```python
from build123d import *

# Parameters (mm, degrees)
SKETCH2_W           = 57.15
SKETCH2_H           = 184.15
BOSS_EXTRUDE1_DEPTH = 6.35
SKETCH3_W           = 44.45
SKETCH3_H           = 6.985
CUT_EXTRUDE1_DEPTH  = 97.616037747
SKETCH4_W           = 6.985
SKETCH4_H           = 50.8
CUT_EXTRUDE2_DEPTH  = 97.616037747


with BuildPart() as part:
    # Sketch2 → Boss-Extrude1 (new body)
    with BuildSketch(Plane.XY):
        Rectangle(SKETCH2_W, SKETCH2_H)
    extrude(amount=BOSS_EXTRUDE1_DEPTH)

    # Sketch3 → Cut-Extrude1 (cut, through all)
    with BuildSketch(Plane.XY.offset(6.35)):
        with Locations((0, 82.2325)):
            Rectangle(SKETCH3_W, SKETCH3_H)
    extrude(amount=-CUT_EXTRUDE1_DEPTH, mode=Mode.SUBTRACT)

    # Sketch4 → Cut-Extrude2 (cut, through all)
    with BuildSketch(Plane.XY.offset(6.35)):
        with Locations((-18.7325, -60.325)):
            Rectangle(SKETCH4_W, SKETCH4_H)
    extrude(amount=-CUT_EXTRUDE2_DEPTH, mode=Mode.SUBTRACT)


solid = part.part
```
Can you work these out from the model? Positions are in its coordinate system, mm. A direction names the side the tool comes from. Give positions to 0.01 mm unless a question says otherwise; leave off trailing zeros. Loops run counter-clockwise (first coordinate to the right, second up) from the corner with the lowest first, then second, coordinate; pieces in that order, holes last. Notation, with made-up numbers: M -31,35.25 L -13,35.25 A28 cw -13,67.25 Z; hole C 0,77.5 d11. An arc over 180 degrees is marked long. Answer in a Markdown table with one row per item.
1. Suppose I cut it at C-C on x = -20. Write out the boundary of the cut face in (y, z) (3 decimals).
Taken from the geometry:
| item | result |
|---|---|
| outline | M -92.075,0 L -85.725,0 L -85.725,6.35 L -92.075,6.35 Z; M -34.925,0 L 78.74,0 L 78.74,6.35 L -34.925,6.35 Z; M 85.725,0 L 92.075,0 L 92.075,6.35 L 85.725,6.35 Z |
2. Which directions (+Z, -Z, +X, -X, +Y, -Y) give clear straight access to the entire face, cutting with the end or side of a thin tool? Please do faces 1 (the flat face through (-15.24, -61, 3)), 2 (the flat face through (28.575, -1, 3)).
Taken from the geometry:
| item | result |
|---|---|
| face 1 | +Z, -Z |
| face 2 | +Z, -Z, +X, +Y, -Y |
3. Suppose I cut it at A-A on x = -6.5. Write out the boundary of the cut face in (y, z) (3 decimals).
Taken from the geometry:
| item | result |
|---|---|
| outline | M -92.075,0 L 78.74,0 L 78.74,6.35 L -92.075,6.35 Z; M 85.725,0 L 92.075,0 L 92.075,6.35 L 85.725,6.35 Z |
4. For pin 1 Ø10 at (x, y) = (-16, -70.5) entering from -Z, with a flat end and sliding along its axis, tell me the tip position at first contact or that it passes through.
Taken from the geometry:
| item | result |
|---|---|
| pin 1 | stops at z = 0 |
5. If I drill on line 1 along Y through (x, z) = (-15.5, 4) (3 decimals); line 2 along Y through (x, z) = (4.5, 3.5) (3 decimals); line 3 along X through (y, z) = (-47, 3.25) (3 decimals), over which ranges is the centre line in solid material (lowest first)?
Taken from the geometry:
| item | result |
|---|---|
| line 1 | y = -92.075 to -85.725, -34.925 to 78.74, 85.725 to 92.075 |
| line 2 | y = -92.075 to 78.74, 85.725 to 92.075 |
| line 3 | x = -28.575 to -22.225, -15.24 to 28.575 |
6. Thinking about a two-plate mould opening in Y: for faces 3 (the flat face through (-22.225, 82, 3)), 4 (the flat face through (0, 92.075, 3)), 5 (the flat face through (0, 1, 6.35)), which applies, released by +Y, released by -Y, zero draft, split by the parting line, or undercut?
Taken from the geometry:
| item | result |
|---|---|
| face 3 | undercut |
| face 4 | released by +Y |
| face 5 | zero draft |
7. Suppose I cut it at B-B on z = 2.75. Write out the boundary of the cut face in (x, y) (3 decimals), plus the area to 3 significant figures.
Taken from the geometry:
| item | result |
|---|---|
| outline | M -28.575,-92.075 L 28.575,-92.075 L 28.575,92.075 L -28.575,92.075 Z; hole M -22.225,-85.725 L -15.24,-85.725 L -15.24,-34.925 L -22.225,-34.925 Z; hole M -22.225,78.74 L 22.225,78.74 L 22.225,85.725 L -22.225,85.725 Z |
| area | 9,860 mm² |
